Build history of the part. All positions in model axes, mm. Give positions to 0.01 mm unless a question says otherwise; leave off trailing zeros. Order: outer loops, then holes, each group sorted by start corner. A loop starts at its lowest first (then second) coordinate and runs counter-clockwise, first axis right, second up. Notation, with made-up numbers: M 11.25,3.25 L 59.25,3.25 A13 cw 59.25,18.25 Z; hole C 9,47 d4. An arc over 180 degrees is marked long. Use CSV: the item, a comma, the result in double quotes. Start each with the question number.
Item 1: Pin check, flat tips, straight feed: P1, Ø1, axis at x = -66.5, y = 3, coming from the +Z side; P2, Ø2, axis at x = -61.5, y = 2.5, coming from the -Z side; P3, Ø2, axis at x = 35.5, y = 2, coming from the -Z side. Stop position of each tip, or through.
Item 2: Wall check: line 1 along X through (y, z) = (1.1, 0); line 2 along Z through (x, y) = (7.5, 1.55); line 3 along X through (y, z) = (0.3, -18). Give the ranges that are in metal, low to high.
Item 3: Band-saw the part on D-D on x = -20. Write the cut outline in (y, z), plus the area to 3 significant figures.
Item 4: Band-saw the part on B-B on x = 41. Write the cut outline in (y, z).
Item 5: Band-saw the part on A-A on z = 0. Write the cut outline in (x, y).
Item 6: Band-saw the part on C-C on y = 0.6. Give the number of separate pieces and of enclosed holes in the cut face, plus the area to 3 significant figures.
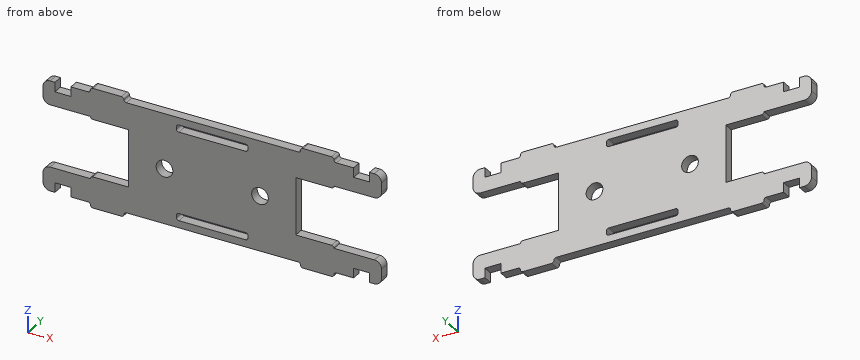
from build123d import *

# Parameters (mm, degrees)
SCHIZZO1_W                   = 30
SCHIZZO1_H                   = 3
SCHIZZO1_R                   = 3.5
ESTRUSIONE_ESTRUSIONE1_DEPTH = 4
RACCORDO1_START              = -1
RACCORDO1_DEPTH              = 6
RACCORDO1_2_DEPTH            = 4
RACCORDO2_R                  = 3
RACCORDO3_R                  = 1
RACCORDO4_R                  = 1


with BuildPart() as part:
    # Schizzo1 → Estrusione-Estrusione1 (new body)
    with BuildSketch(Plane(origin=(0, 0, 0), x_dir=(1, 0, 0), z_dir=(0, 1, 0))):
        Polygon((-65.9, 19), (-65.9, 23), (-70.9, 23), (-70.9, 13), (-51, 13), (-51, 12), (-35, 12), (-35, -12), (-51, -12), (-51, -13), (-70.9, -13), (-70.9, -23), (-65.9, -23), (-65.9, -19), (-59.2, -19), (-59.2, -23), (-51, -23), (-51, -25), (-37, -25), (-37, -23), (37, -23), (37, -25), (51, -25), (51, -23), (59.2, -23), (59.2, -19), (65.9, -19), (65.9, -23), (70.9, -23), (70.9, -13), (51, -13), (51, -12), (35, -12), (35, 12), (51, 12), (51, 13), (70.9, 13), (70.9, 23), (65.9, 23), (65.9, 19), (59.2, 19), (59.2, 23), (51, 23), (51, 25), (37, 25), (37, 23), (-37, 23), (-37, 25), (-51, 25), (-51, 23), (-59.2, 23), (-59.2, 19), align=None)
        with Locations((0, -18.5)):
            Rectangle(SCHIZZO1_W, SCHIZZO1_H, mode=Mode.SUBTRACT)
        with Locations(Location((20, 0, 0), (0, 0, 270))):
            Circle(SCHIZZO1_R, mode=Mode.SUBTRACT)
        with Locations((0, 18.5)):
            Rectangle(SCHIZZO1_W, SCHIZZO1_H, mode=Mode.SUBTRACT)
        with Locations(Location((-20, 0, 0), (0, 0, 270))):
            Circle(SCHIZZO1_R, mode=Mode.SUBTRACT)
    extrude(amount=ESTRUSIONE_ESTRUSIONE1_DEPTH)

    # Raccordo1: read off the stored shape, not the designer's step
    # Raccordo1 outline → Raccordo1 (cut)
    with BuildSketch(Plane(origin=(0, 0, 0), x_dir=(1, 0, 0), z_dir=(0, 1, 0)).offset(RACCORDO1_START)):
        with BuildLine():
            Line((51, -25), (51, -24))
            ThreePointArc((51, -24), (50.707106781, -24.707106781), (50, -25))
            Line((50, -25), (51, -25))
        make_face()
        with BuildLine():
            Line((-51, -25), (-50, -25))
            ThreePointArc((-50, -25), (-50.707106781, -24.707106781), (-51, -24))
            Line((-51, -24), (-51, -25))
        make_face()
        with BuildLine():
            Line((-37, -25), (-37, -24))
            ThreePointArc((-37, -24), (-37.292893219, -24.707106781), (-38, -25))
            Line((-38, -25), (-37, -25))
        make_face()
        with BuildLine():
            Line((37, -25), (38, -25))
            ThreePointArc((38, -25), (37.292893219, -24.707106781), (37, -24))
            Line((37, -24), (37, -25))
        make_face()
        with BuildLine():
            Line((37, 25), (37, 24))
            ThreePointArc((37, 24), (37.292893219, 24.707106781), (38, 25))
            Line((38, 25), (37, 25))
        make_face()
        with BuildLine():
            ThreePointArc((-51, 24), (-50.707106781, 24.707106781), (-50, 25))
            Line((-50, 25), (-51, 25))
            Line((-51, 25), (-51, 24))
        make_face()
        with BuildLine():
            ThreePointArc((-38, 25), (-37.292893219, 24.707106781), (-37, 24))
            Line((-37, 24), (-37, 25))
            Line((-37, 25), (-38, 25))
        make_face()
        with BuildLine():
            Line((51, 25), (50, 25))
            ThreePointArc((50, 25), (50.707106781, 24.707106781), (51, 24))
            Line((51, 24), (51, 25))
        make_face()
    extrude(amount=RACCORDO1_DEPTH, mode=Mode.SUBTRACT)

    # Raccordo1 2 outline → Raccordo1 2 (add)
    with BuildSketch(Plane(origin=(0, 0, 0), x_dir=(1, 0, 0), z_dir=(0, 1, 0))):
        with BuildLine():
            Line((51, -23), (51, -24))
            ThreePointArc((51, -24), (51.292893219, -23.292893219), (52, -23))
            Line((52, -23), (51, -23))
        make_face()
        with BuildLine():
            ThreePointArc((-52, -23), (-51.292893219, -23.292893219), (-51, -24))
            Line((-51, -24), (-51, -23))
            Line((-51, -23), (-52, -23))
        make_face()
        with BuildLine():
            ThreePointArc((-37, -24), (-36.707106781, -23.292893219), (-36, -23))
            Line((-36, -23), (-37, -23))
            Line((-37, -23), (-37, -24))
        make_face()
        with BuildLine():
            ThreePointArc((36, -23), (36.707106781, -23.292893219), (37, -24))
            Line((37, -24), (37, -23))
            Line((37, -23), (36, -23))
        make_face()
        with BuildLine():
            Line((37, 23), (37, 24))
            ThreePointArc((37, 24), (36.707106781, 23.292893219), (36, 23))
            Line((36, 23), (37, 23))
        make_face()
        with BuildLine():
            Line((-51, 23), (-51, 24))
            ThreePointArc((-51, 24), (-51.292893219, 23.292893219), (-52, 23))
            Line((-52, 23), (-51, 23))
        make_face()
        with BuildLine():
            Line((-37, 23), (-36, 23))
            ThreePointArc((-36, 23), (-36.707106781, 23.292893219), (-37, 24))
            Line((-37, 24), (-37, 23))
        make_face()
        with BuildLine():
            ThreePointArc((52, 23), (51.292893219, 23.292893219), (51, 24))
            Line((51, 24), (51, 23))
            Line((51, 23), (52, 23))
        make_face()
    extrude(amount=RACCORDO1_2_DEPTH)

    # Raccordo2
    raccordo2_edges = [part.edges().sort_by_distance(p)[0] for p in [
        (70.9, 2, 13),
        (70.9, 2, 23),
        (-70.9, 2, 23),
        (-70.9, 2, 13),
        (-70.9, 2, -13),
        (-70.9, 2, -23),
        (70.9, 2, -23),
        (70.9, 2, -13),
    ]]
    fillet(raccordo2_edges, radius=RACCORDO2_R)

    # Raccordo3
    raccordo3_edges = [part.edges().sort_by_distance(p)[0] for p in [
        (51, 2, -12),
        (51, 2, 12),
        (-51, 2, 12),
        (-51, 2, -12),
    ]]
    fillet(raccordo3_edges, radius=RACCORDO3_R - 0.0001)  # a hair under: the kernel refuses the full size

    # Raccordo4
    raccordo4_edges = [part.edges().sort_by_distance(p)[0] for p in [
        (15, 2, 17),
        (-15, 2, 17),
        (-15, 2, 20),
        (15, 2, 20),
        (15, 2, -20),
        (-15, 2, -20),
        (-15, 2, -17),
        (15, 2, -17),
    ]]
    fillet(raccordo4_edges, radius=RACCORDO4_R)


solid = part.part
Model answer:
1,P1,"stops at z = 23"
1,P2,"stops at z = -19"
1,P3,"stops at z = -23.13"
2,line 1,"x = -35 to -23.5, -16.5 to 16.5, 23.5 to 35"
2,line 2,"z = -23 to -20, -17 to 17, 20 to 23"
2,line 3,"x = -70.9 to -15, 15 to 70.9"
3,outline,"M 0,-23 L 4,-23 L 4,-3.5 L 0,-3.5 Z; M 0,3.5 L 4,3.5 L 4,23 L 0,23 Z"
3,area,"156 mm^2"
4,outline,"M 0,-25 L 4,-25 L 4,-12 L 0,-12 Z; M 0,12 L 4,12 L 4,25 L 0,25 Z"
5,outline,"M -35,0 L -23.5,0 L -23.5,4 L -35,4 Z; M -16.5,0 L 16.5,0 L 16.5,4 L -16.5,4 Z; M 23.5,0 L 35,0 L 35,4 L 23.5,4 Z"
6,separate pieces,"1"
6,enclosed holes,"4"
6,area,"4,450 mm^2"
